```python
from build123d import *

# Parameters (mm, degrees)
F0_R           = 10.5
F1_DEPTH       = 10
F3_R           = 17
F3_R_2         = 2
F3_R_3         = 9.1303140993
F4_DEPTH       = 4
F5_D           = 4
F5_DEPTH       = 10
F5_CSINK_D     = 6.5
F5_CSINK_ANGLE = 90
F5_TIP         = 1.2017212381
F7_DEPTH       = 8


with BuildPart() as f1:
    # F0 (on Top) → F1 (new body)
    with BuildSketch(Plane.XY):
        Circle(F0_R)
        with BuildLine():
            ThreePointArc((-5, 0), (-4.1213203436, 2.1213203436), (-2, 3))
            Line((-2, 3), (2, 3))
            ThreePointArc((2, 3), (4.1213203436, 2.1213203436), (5, 0))
            ThreePointArc((5, 0), (4.1213203436, -2.1213203436), (2, -3))
            Line((2, -3), (-2, -3))
            ThreePointArc((-2, -3), (-4.1213203436, -2.1213203436), (-5, 0))
        make_face(mode=Mode.SUBTRACT)
    extrude(amount=-F1_DEPTH)

    # F3 (on offset) → F4 (join)
    with BuildSketch(Plane(origin=(0, 0, -10), x_dir=(1, 0, 0), z_dir=(0, 0, -1))):
        Circle(F3_R)
        with Locations((0, -13.75)):
            Circle(F3_R_2, mode=Mode.SUBTRACT)
        Circle(F3_R_3, mode=Mode.SUBTRACT)
        with Locations((0, 13.75)):
            Circle(F3_R_2, mode=Mode.SUBTRACT)
    extrude(amount=-F4_DEPTH)

    # F5
    with Locations(Plane(origin=(0, 0, -10), x_dir=(1, 0, 0), z_dir=(0, 0, -1))):
        with Locations((0, 13.75), (0, -13.75)):
            CounterSinkHole(F5_D / 2, F5_CSINK_D / 2, depth=F5_DEPTH, counter_sink_angle=F5_CSINK_ANGLE)
            with Locations((0, 0, -(F5_DEPTH + F5_TIP / 2))):  # 118° drill point
                Cone(0, F5_D / 2, F5_TIP, mode=Mode.SUBTRACT)

    # F6 (on face) → F7 (cut)
    with BuildSketch(Plane.XY):
        with BuildLine():
            Line((2, 5), (-2, 5))
            ThreePointArc((-2, 5), (-5.5355339059, 3.5355339059), (-7, 0))
            ThreePointArc((-7, 0), (-5.5355339059, -3.5355339059), (-2, -5))
            Line((-2, -5), (2, -5))
            ThreePointArc((2, -5), (5.5355339059, -3.5355339059), (7, 0))
            ThreePointArc((7, 0), (5.5355339059, 3.5355339059), (2, 5))
        make_face()
        with BuildLine():
            Line((2, -3), (-2, -3))
            ThreePointArc((-2, -3), (-5, 0), (-2, 3))
            Line((-2, 3), (2, 3))
            ThreePointArc((2, 3), (5, 0), (2, -3))
        make_face(mode=Mode.SUBTRACT)
    extrude(amount=-F7_DEPTH, mode=Mode.SUBTRACT)


solid = f1.part
```
Input: part model. Units: mm. Frame: model coordinates. A direction names the side the tool comes from. Coordinates: 2 decimals unless noted, no trailing zeros. Loops run counter-clockwise (first coordinate to the right, second up) from the corner with the lowest first, then second, coordinate; pieces in that order, holes last.
Q1. Section D-D, the plane z = -4.25. Return the cut outline in (x, y), and give its area (3 significant figures).
Results are:
outline: circle Ø21 at (0, 0); hole (-2, -5) - (2, -5) arc R5 ccw to (2, 5) - (-2, 5) arc R5 ccw to start
area: 228 mm2
Q2. Line query: line 1 along Y through (x, z) = (0, -8.05); line 2 along Y through (x, z) = (0, -6.7); line 3 along Z through (x, y) = (7.5, 11). Output: solid intervals per line, ascending.
Results are:
line 1: y = -17 to -15.75, -11.75 to -3, 3 to 11.75, 15.75 to 17
line 2: y = -17 to -15.75, -11.75 to -5, 5 to 11.75, 15.75 to 17
line 3: z = -10 to -6
Q3. Section C-C, the plane y = 13.75. Return the cut outline in (x, z).
Results are:
outline: (-10, -10) - (-3.25, -10) - (-2, -8.75) - (-2, -6) - (-10, -6) - close; (2, -8.75) - (3.25, -10) - (10, -10) - (10, -6) - (2, -6) - close
Q4. Section B-B, the plane x = 4. Return the cut outline in (y, z).
Results are:
outline: (-16.52, -10) - (-2.24, -10) - (-2.24, -8) - (-4.58, -8) - (-4.58, 0) - (-9.71, 0) - (-9.71, -6) - (-16.52, -6) - close; (2.24, -10) - (16.52, -10) - (16.52, -6) - (9.71, -6) - (9.71, 0) - (4.58, 0) - (4.58, -8) - (2.24, -8) - close
Q5. Section A-A, the plane z = -7. Return the cut outline in (x, y), and give its area (3 significant figures).
Results are:
outline: circle Ø34 at (0, 0); hole circle Ø4 at (0, -13.75); hole (-2, -5) - (2, -5) arc R5 ccw to (2, 5) - (-2, 5) arc R5 ccw to start; hole circle Ø4 at (0, 13.75)
area: 764 mm2
Q6. Mould query, pull axis Y, two halves, no side actions, for faces 4 (the flat face through (7.3, -7.8, -6)), 5 (the cylindrical face through (0.923, 15.524, -7.394)), 6 (the cylindrical face through (10, 3.2, -3)). Classes: +Y half, -Y half, draft (parallel to the pull), parting line (faces both ways), or undercut.
Results are:
face 4: draft
face 5: undercut
face 6: parting line
Q7. Set-up query: faces 1 (the flat face through (-0.1, 3.4, -8)), 2 (the flat face through (0, 3, -9)), 3 (the conical face through (0, -16, -9)). Return all of +Z, -Z, +X, -X, +Y, -Y with unobstructed straight access to the full face (end or side cutting, diameter ignored); none if empty.
Results are:
face 1: +Z
face 2: +Z, -Z
face 3: -Z
Q8. Contact query for flat-ended pins moving along their axis: pin 1 (5 mm diameter, centred on x = 0, y = -13.75, fed in from +Z); pin 2 (3 mm diameter, centred on x = 0.5, y = -1, fed in from +Z); pin 3 (1 mm diameter, centred on x = 11, z = -9, fed in from +Y); pin 4 (1 mm diameter, centred on x = -4, z = -7.5, fed in from -Y). Output: stop coordinate, or through.
Results are:
pin 1: stops at z = -6
pin 2: passes through
pin 3: stops at y = 13.37
pin 4: stops at y = -16.64
